For this review, take the finished solid that the model builds, in its own axes (mm). Round coordinates to 2 decimals unless told otherwise and drop trailing zeros. Order: outer loops, then holes, each group sorted by start corner. A loop starts at its lowest first (then second) coordinate and runs counter-clockwise, first axis right, second up.
```python
from build123d import *

# Parameters (mm, degrees)
SKETCH1_W               = 81.3
SKETCH1_H               = 51
BOSS_EXTRUDE1_DEPTH     = 1.5
FILLET1_R               = 2
CUT_EXTRUDE1_DEPTH      = 96.984061177
CUT_EXTRUDE1_DEPTH_BACK = 96.984061177
SKETCH2_R               = 1.75


with BuildPart() as part:
    # Sketch1 → Boss-Extrude1 (new body)
    with BuildSketch(Plane(origin=(0, 0, 0), x_dir=(1, 0, 0), z_dir=(0, 1, 0))):
        with Locations((40.65, 25.5)):
            Rectangle(SKETCH1_W, SKETCH1_H)
    extrude(amount=BOSS_EXTRUDE1_DEPTH)

    # Fillet1
    fillet1_edges = [part.edges().sort_by_distance(p)[0] for p in [
        (0, 0.75, -51),
        (81.3, 0.75, -51),
        (81.3, 0.75, 0),
        (0, 0.75, 0),
    ]]
    fillet(fillet1_edges, radius=FILLET1_R)

    # Sketch2 → Cut-Extrude1 (cut, two sides: drawn at the far end of the back side and taken through both)
    with BuildSketch(Plane(origin=(0, 1.5, 0), x_dir=(1, 0, 0), z_dir=(0, 1, 0)).offset(-CUT_EXTRUDE1_DEPTH_BACK)):
        with Locations(Location((3.85, 25.5, 0), (0, 0, 270))):
            Circle(SKETCH2_R)
        with Locations(Location((77.45, 25.5, 0), (0, 0, 270))):
            Circle(SKETCH2_R)
    extrude(amount=CUT_EXTRUDE1_DEPTH + CUT_EXTRUDE1_DEPTH_BACK, mode=Mode.SUBTRACT)


solid = part.part
```
Q1. Wall thickness on line 1 (X direction, y = 0.75, z = -25.5); line 2 (Z direction, x = 3.85, y = 0.5); line 3 (X direction, y = 0.8, z = -26.5): over which ranges is each line inside the solid? List them lowest first.
Q2. Take a section at A-A, the plane x = 3.85. State the section outline as (y, z) points, plus the area to 4 significant figures.
Q3. Take a section at B-B, the plane z = -25.5. State the section outline as (x, y) points, plus the area to 3 significant figures.
Q4. Mouldability with a two-part tool opening along Z and no side actions: class faces 1 (the face through (40, 0, -26)), 2 (the face through (0.57, 0.76, -50.4)), 3 (the face through (40, 1, 0)), 4 (the face through (75.74, 0.74, -25.88)) as +Z half, -Z half, draft (parallel to the pull), parting line (faces both ways), or undercut.
Q5. Clearance check with a flat-ended pin moving along its axis: pin 1 (4 mm diameter, centred on x = 32, z = -31, fed in from -Y). State where the tip first meets the part, or that it passes through.
Working result:
1. line 1: x = 0 to 2.1, 5.6 to 75.7, 79.2 to 81.3
1. line 2: z = -51 to -27.25, -23.75 to 0
1. line 3: x = 0 to 2.41, 5.29 to 76.01, 78.89 to 81.3
2. outline: (0, -51) - (1.5, -51) - (1.5, -27.25) - (0, -27.25) - close; (0, -23.75) - (1.5, -23.75) - (1.5, 0) - (0, 0) - close
2. area: 71.25 mm2
3. outline: (0, 0) - (2.1, 0) - (2.1, 1.5) - (0, 1.5) - close; (5.6, 0) - (75.7, 0) - (75.7, 1.5) - (5.6, 1.5) - close; (79.2, 0) - (81.3, 0) - (81.3, 1.5) - (79.2, 1.5) - close
3. area: 111 mm2
4. face 1: draft
4. face 2: -Z half
4. face 3: +Z half
4. face 4: undercut
5. pin 1: stops at y = 0
